Geometry check sheet. Reference: the model listing, model coordinates, mm. A direction names the side the tool comes from. Give positions to 0.01 mm unless a question says otherwise; leave off trailing zeros. Order: outer loops, then holes, each group sorted by start corner. A loop starts at its lowest first (then second) coordinate and runs counter-clockwise, first axis right, second up. Notation, with made-up numbers: M -19,70 L 35,70 A28 cw 35,105 Z; hole C 14,-2 d8. An arc over 180 degrees is marked long. One line per question, with ' | ' between items. Start each with the question number.
Autodesk Inventor part; units mm, degrees
ref_plane "YZ Plane" through (0, 0, 0) normal (1, 0, 0) x (0, 1, 0)
ref_plane "XZ Plane" through (0, 0, 0) normal (0, 1, 0) x (-1, 0, 0)
ref_plane "XY Plane" through (0, 0, 0) normal (0, 0, 1) x (1, 0, 0)
sketch "Skizze1" plane through (0, 0, 0) normal (0, 0, 1) x (1, 0, 0)
  line L0 (0, 0) -> (6, 0)
  line L1 (6, 0) -> (6, 16.5)
  line L2 (6, 16.5) -> (7, 16.5)
  line L3 (7, 16.5) -> (7, 17.5)
  line L4 (7, 17.5) -> (5.8187, 17.8052)
  line L5 (5.8187, 17.8052) -> (5.9982, 18.5)
  line L6 (5.9982, 18.5) -> (0, 18.5)
  line L7 (0, 18.5) -> (0, 0)
  point P0 (6.5, 16.5)
  dimension "d0" = 6
  dimension "d1" = 16.5
  dimension "d2" = 7
  dimension "d3" = 1
  dimension "d4" = 2
revolve "Umdrehung1" add sketch "Skizze1" angle 360 about axis through (0, 18.5, 0) along (0, -1, 0)
sketch "Skizze2" plane through (0, 0, 0) normal (0, -1, 0) x (1, 0, 0)
  line L0 (-5.3128, 0.8351) -> (5.1112, 0.8351)
  line L1 (5.1112, 0.8351) -> (5.1112, -1.0078)
  line L2 (5.1112, -1.0078) -> (-5.3128, -1.0078)
  line L3 (-5.3128, -1.0078) -> (-5.3128, 0.8351)
  point P0 (0, 0)
extrude "Extrusion1" add sketch "Skizze2" along normal blind 4.5
properties part number "Knopf"
Item 1: Cross-section at A-A, the plane x = 0. Record the cut outline in (y, z).
Item 2: Set-up check for faces 1 (the flat face through (5.111, -2, 0)), 2 (the flat face through (0, -2, 0.835)), 3 (the cylindrical face through (-6, 8, 0)), 4 (the flat face through (-5.313, -2, 0)), 5 (the flat face through (0, -2, -1.008)): record each of +Z, -Z, +X, -X, +Y, -Y from which the full face is reachable in a straight line by a thin tool's end or side.
Item 3: Cross-section at C-C, the plane z = 0. Record the cut outline in (x, y), plus the area to 3 significant figures.
Item 4: Depth check by flat-ended pin: pin 1 (3 mm diameter, centred on x = 2, y = 13.5, fed in from -Z); pin 2 (0.9 mm diameter, centred on y = -2, z = 0, fed in from -X); pin 3 (2 mm diameter, centred on x = -5, y = 14, fed in from +Z). Enter the tip coordinate at first touch or a pass-through.
Item 5: Cross-section at B-B, the plane y = 8.5. Record the cut outline in (x, z), plus the area to 3 significant figures.
Item 6: Material ranges on line 1 along Z through (x, y) = (2.5, -1); line 2 along Z through (x, y) = (0, 14.5); line 3 along X through (y, z) = (-2.5, 0.75), recorded low to high.
Item 7: Cross-section at D-D, the plane y = -0.5. Record the cut outline in (x, z), plus the area to 3 significant figures.
Outcome:
1) outline: M -4.5,-1.01 L 0,-1.01 L 0,-6 L 16.5,-6 L 16.5,-7 L 17.5,-7 L 17.81,-5.82 L 18.5,-6 L 18.5,6 L 17.81,5.82 L 17.5,7 L 16.5,7 L 16.5,6 L 0,6 L 0,0.84 L -4.5,0.84 Z
2) face 1: +Z, -Z, +X, -Y | face 2: +Z, +X, -X, -Y | face 3: -Y | face 4: +Z, -Z, -X, -Y | face 5: -Z, +X, -X, -Y
3) outline: M -7,16.5 L -6,16.5 L -6,0 L -5.31,0 L -5.31,-4.5 L 5.11,-4.5 L 5.11,0 L 6,0 L 6,16.5 L 7,16.5 L 7,17.5 L 5.82,17.81 L 6,18.5 L -6,18.5 L -5.82,17.81 L -7,17.5 Z | area: 271 mm²
4) pin 1: stops at z = -5.98 | pin 2: stops at x = -5.31 | pin 3: stops at z = 4.47
5) outline: C 0,0 d12 | area: 113 mm²
6) line 1: z = -1.01 to 0.84 | line 2: z = -6 to 6 | line 3: x = -5.31 to 5.11
7) outline: M -5.31,-1.01 L 5.11,-1.01 L 5.11,0.84 L -5.31,0.84 Z | area: 19.2 mm²
